The figure shows three views and two pictorial views of one solid part (mm, origin at its lowest corner). Answer the questions. A direction names the side the tool comes from. Round coordinates to 2 decimals unless told otherwise and drop trailing zeros. Order: outer loops, then holes, each group sorted by start corner. A loop starts at its lowest first (then second) coordinate and runs counter-clockwise, first axis right, second up. Notation, with made-up numbers: (-37.75, 87.25) -> (-33.75, 87.25) arc R28 ccw to (-33.75, 117.25) -> close; hole circle Ø7 at (5.25, -20.5). An arc over 180 degrees is marked (long way). One line per item, written item: value. Start each with the question number.
1. Section A-A (x = 1.5) is taken. Give the vertices of the cut face in (y, z), then the cut area to 3 significant figures.
2. The mould has two halves that part along X. Classify the marked faces 1, 2 and 3: released by +X, released by -X, zero draft, split by the parting line, or undercut.
3. Consider line 1 (Y direction, x = 2, z = 3.5); line 2 (Y direction, x = 3.25, z = 2); line 3 (X direction, y = 6.5, z = 5). Determine where each line is inside the solid, lowest interval first.
4. Flat-ended cylindrical pins translate along their axes: pin 1 Ø2 at (x, y) = (5.5, 3) entering from -Z; pin 2 Ø1.5 at (x, z) = (2.5, 4.5) entering from +Y; pin 3 Ø2 at (y, z) = (1.5, 5) entering from -X; pin 4 Ø1.5 at (x, y) = (6, 1.5) entering from -Z. Find the tip coordinate at first contact, or state that the pin passes through.
5. For the marked faces 4 and 5, determine the directions among +Z, -Z, +X, -X, +Y, -Y from which every point of the face is accessible in a straight line to the end or side of a thin tool.
6. Section B-B (x = 6.25) is taken. Give the vertices of the cut face in (y, z).
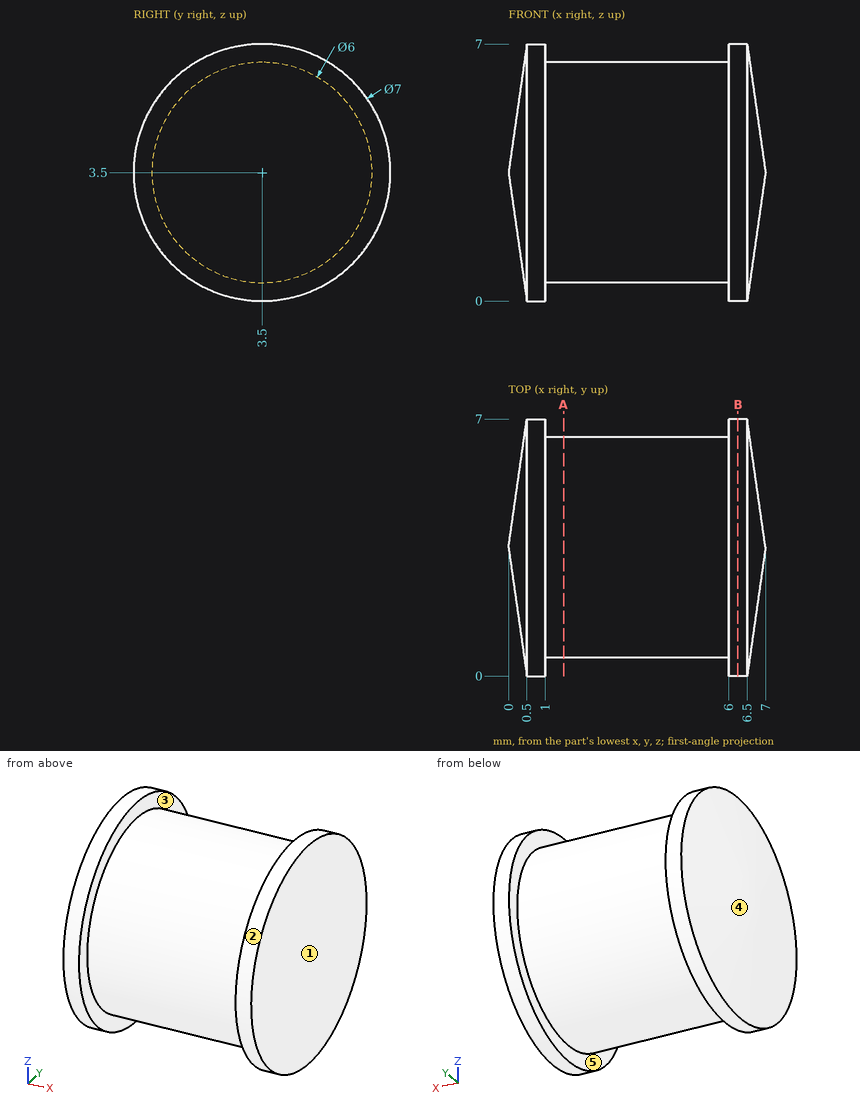
Answer:
1. outline: circle Ø6 at (3.5, 3.5)
1. area: 28.3 mm^2
2. face 1: released by +X
2. face 2: zero draft
2. face 3: undercut
3. line 1: 0.5 to 6.5
3. line 2: 0.9 to 6.1
3. line 3: 0.48 to 1, 6 to 6.52
4. pin 1: z = 0
4. pin 2: y = 6.49
4. pin 3: x = 0.21
4. pin 4: z = 0.23
5. face 4: -X
5. face 5: none
6. outline: circle Ø7 at (3.5, 3.5)
